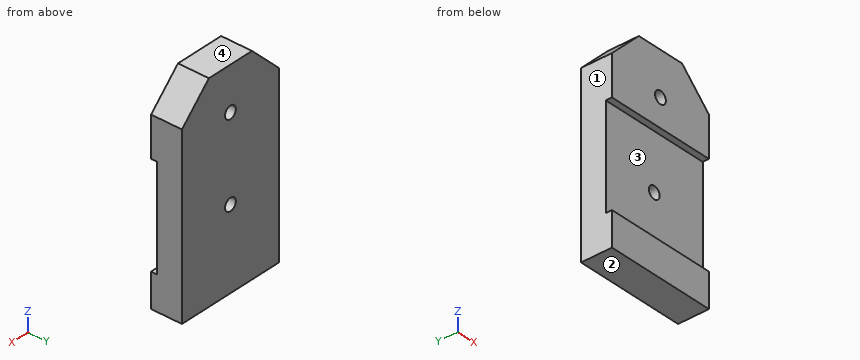
from build123d import *

# Parameters (mm, degrees)
F1_DEPTH = 5
F2_W     = 18
F2_H     = 16.5
F3_DEPTH = 1
F4_R     = 1
F5_DEPTH = 5.001
F6_R     = 1
F7_DEPTH = 4.001


with BuildPart() as f1:
    # F0 (on Front) → F1 (new body)
    with BuildSketch(Plane.XZ):
        Polygon((0, 28.5), (0, 0), (18, 0), (18, 28.5), (13, 33.5), (5, 33.5), align=None)
    extrude(amount=F1_DEPTH)

    # F2 (on face) → F3 (cut)
    with BuildSketch(Plane.XZ.offset(5)):
        with Locations((9, 13.75)):
            Rectangle(F2_W, F2_H)
    extrude(amount=-F3_DEPTH, mode=Mode.SUBTRACT)

    # F4 (on face) → F5 (cut, through all)
    with BuildSketch(Plane.XZ.offset(5)):
        with Locations((9, 26.5)):
            Circle(F4_R)
    extrude(amount=-F5_DEPTH, mode=Mode.SUBTRACT)

    # F6 (on face) → F7 (cut, through all)
    with BuildSketch(Plane.XZ.offset(4)):
        with Locations((9, 13)):
            Circle(F6_R)
    extrude(amount=-F7_DEPTH, mode=Mode.SUBTRACT)


solid = f1.part
For this review, take the finished solid that the model builds, in its own axes (mm). Face numbers are marked on the shaded views. Round coordinates to 2 decimals unless told otherwise and drop trailing zeros. Loops run counter-clockwise (first coordinate to the right, second up) from the corner with the lowest first, then second, coordinate; pieces in that order, holes last. Notation, with made-up numbers: (22.25, -39) - (50.25, -39) arc R24 ccw to (50.25, -19) - close; hole circle Ø4 at (53, -11). An arc over 180 degrees is marked (long way). Answer as CSV lines item,"result".
(1) Insertion check: P1, Ø3, axis at x = 6, y = -2, coming from the -Z side; P2, Ø1.6, axis at x = 9, z = 26.5, coming from the +Y side (3 decimals); P3, Ø5, axis at x = 9, z = 13, coming from the -Y side. Each pin has a flat end and moves straight along its axis. Give the tip position at first contact, or say it passes through.
Checked values:
P1,"stops at z = 0"
P2,"passes through"
P3,"stops at y = -4"
(2) Consider section A-A on x = 9. Give the boundary of the cut face in (y, z).
Checked values:
outline,"(-5, 0) - (0, 0) - (0, 12) - (-4, 12) - (-4, 5.5) - (-5, 5.5) - close; (-5, 22) - (-4, 22) - (-4, 14) - (0, 14) - (0, 25.5) - (-5, 25.5) - close; (-5, 27.5) - (0, 27.5) - (0, 33.5) - (-5, 33.5) - close"
(3) Wall thickness on line 1 (Z direction, x = 9, y = -3.6); line 2 (Z direction, x = 9.75, y = -1); line 3 (Z direction, x = 5, y = -4.15): over which ranges is each line inside the solid? List them lowest first.
Checked values:
line 1,"z = 0 to 12, 14 to 25.5, 27.5 to 33.5"
line 2,"z = 0 to 12.34, 13.66 to 25.84, 27.16 to 33.5"
line 3,"z = 0 to 5.5, 22 to 33.5"
(4) Consider section B-B on y = -1.1. Give the boundary of the cut face in (x, z).
Checked values:
outline,"(0, 0) - (18, 0) - (18, 28.5) - (13, 33.5) - (5, 33.5) - (0, 28.5) - close; hole circle Ø2 at (9, 13); hole circle Ø2 at (9, 26.5)"
(5) Consider section D-D on x = 3.5. Give the boundary of the cut face in (y, z), then the cut area to 4 significant figures.
Checked values:
outline,"(-5, 0) - (0, 0) - (0, 32) - (-5, 32) - (-5, 22) - (-4, 22) - (-4, 5.5) - (-5, 5.5) - close"
area,"143.5 mm2"
(6) Mouldability with a two-part tool opening along Z and no side actions: class the marked faces 1, 2, 3 and 4 as +Z half, -Z half, draft (parallel to the pull), parting line (faces both ways), or undercut.
Checked values:
face 1,"draft"
face 2,"-Z half"
face 3,"undercut"
face 4,"+Z half"
(7) Consider section C-C on z = 26.5. Give the boundary of the cut face in (x, y).
Checked values:
outline,"(0, -5) - (8, -5) - (8, 0) - (0, 0) - close; (10, -5) - (18, -5) - (18, 0) - (10, 0) - close"
